Build history of the part. All positions in model axes, mm. Face numbers are marked on the shaded views. A direction names the side the tool comes from. Give positions to 0.01 mm unless a question says otherwise; leave off trailing zeros. Write each loop counter-clockwise with the first axis right and the second up, starting at its lowest first coordinate (ties: lowest second). Pieces come first, ordered by that corner, then holes. Notation, with made-up numbers: M 4.5,44 L 10.5,44 A19 cw 10.5,56 Z; hole C 77,66.5 d7. An arc over 180 degrees is marked long. One line per item, written item: value. Start each with the question number.
from build123d import *

# Parameters (mm, degrees)
SKETCH1_W           = 38
SKETCH1_H           = 30
SKETCH1_W_2         = 35
SKETCH1_H_2         = 27.631578948
BOSS_EXTRUDE1_DEPTH = 28.84
FILLET1_R           = 1
SKETCH2_W           = 35
SKETCH2_H           = 27.631578948
BOSS_EXTRUDE2_DEPTH = 3
SKETCH3_W           = 36.5
SKETCH3_H           = 28.815789474
CUT_EXTRUDE1_DEPTH  = 36.407705376
FILLET2_R           = 1


with BuildPart() as part:
    # Sketch1 → Boss-Extrude1 (new body)
    with BuildSketch(Plane.XY):
        Rectangle(SKETCH1_W, SKETCH1_H)
        Rectangle(SKETCH1_W_2, SKETCH1_H_2, mode=Mode.SUBTRACT)
    extrude(amount=BOSS_EXTRUDE1_DEPTH)

    # Fillet1
    fillet1_edges = [part.edges().sort_by_distance(p)[0] for p in [
        (19, 0, 28.84),
        (0, 15, 28.84),
        (-19, 0, 28.84),
        (0, -15, 28.84),
    ]]
    fillet(fillet1_edges, radius=FILLET1_R)

    # Sketch2 → Boss-Extrude2 (add)
    with BuildSketch(Plane(origin=(0, 0, 0), x_dir=(-1, 0, 0), z_dir=(0, 0, -1))):
        Rectangle(SKETCH2_W, SKETCH2_H)
    extrude(amount=-BOSS_EXTRUDE2_DEPTH)

    # Sketch3 → Cut-Extrude1 (cut, through all)
    with BuildSketch(Plane(origin=(0, 0, 3), x_dir=(-1, 0, 0), z_dir=(0, 0, -1))):
        with Locations((-0.75, -0.592105263)):
            Rectangle(SKETCH3_W, SKETCH3_H)
    extrude(amount=-CUT_EXTRUDE1_DEPTH, mode=Mode.SUBTRACT)

    # Fillet2
    # the kernel refuses this fillet: 1 mm, written as the material it takes off along each edge
    with BuildSketch(Plane(origin=(-18, -14, 27.84), x_dir=(-1, 0, 0), z_dir=(0, -1, 0))) as fillet2_piece_1_section:
        Polygon((0, 0), (FILLET2_R * 1.02, 0), (FILLET2_R * 1.02, -FILLET2_R * 1.02), (0, -FILLET2_R * 1.02), align=None)
    fillet2_piece_1 = extrude(amount=FILLET2_R * 1.02, mode=Mode.PRIVATE)
    fillet2_piece_1 = fillet2_piece_1 - Plane(origin=(-18, -14, 27.84), x_dir=(0.7071067811865475, 0, -0.7071067811865475), z_dir=(0, -1, 0)) * Sphere(FILLET2_R, mode=Mode.PRIVATE)
    add(fillet2_piece_1, mode=Mode.SUBTRACT)
    with BuildSketch(Plane(origin=(-18, 14, 27.84), x_dir=(-1, 0, 0), z_dir=(0, 1, 0))) as fillet2_piece_2_section:
        Polygon((0, 0), (FILLET2_R * 1.02, 0), (FILLET2_R * 1.02, FILLET2_R * 1.02), (0, FILLET2_R * 1.02), align=None)
    fillet2_piece_2 = extrude(amount=FILLET2_R * 1.02, mode=Mode.PRIVATE)
    fillet2_piece_2 = fillet2_piece_2 - Plane(origin=(-18, 14, 27.84), x_dir=(0.7071067811865475, 0, -0.7071067811865475), z_dir=(0, 1, 0)) * Sphere(FILLET2_R, mode=Mode.PRIVATE)
    add(fillet2_piece_2, mode=Mode.SUBTRACT)
    with BuildSketch(Plane(origin=(18, 14, 27.84), x_dir=(0, 1, 0), z_dir=(1, 0, 0))) as fillet2_piece_3_section:
        Polygon((0, 0), (FILLET2_R * 1.02, 0), (FILLET2_R * 1.02, FILLET2_R * 1.02), (0, FILLET2_R * 1.02), align=None)
    fillet2_piece_3 = extrude(amount=FILLET2_R * 1.02, mode=Mode.PRIVATE)
    fillet2_piece_3 = fillet2_piece_3 - Plane(origin=(18, 14, 27.84), x_dir=(0, -0.7071067811865475, -0.7071067811865475), z_dir=(1, 0, 0)) * Sphere(FILLET2_R, mode=Mode.PRIVATE)
    add(fillet2_piece_3, mode=Mode.SUBTRACT)
    with BuildSketch(Plane(origin=(18, -14, 1), x_dir=(1, 0, 0), z_dir=(0, -1, 0))) as fillet2_piece_4_section:
        Polygon((0, 0), (FILLET2_R * 1.02, 0), (FILLET2_R * 1.02, -FILLET2_R * 1.02), (0, -FILLET2_R * 1.02), align=None)
    fillet2_piece_4 = extrude(amount=FILLET2_R * 1.02, mode=Mode.PRIVATE)
    fillet2_piece_4 = fillet2_piece_4 - Plane(origin=(18, -14, 1), x_dir=(-0.7071067811865475, 0, 0.7071067811865475), z_dir=(0, -1, 0)) * Sphere(FILLET2_R, mode=Mode.PRIVATE)
    add(fillet2_piece_4, mode=Mode.SUBTRACT)
    with BuildSketch(Plane(origin=(18, -14, 2), x_dir=(1, 0, 0), z_dir=(0, -1, 0))) as fillet2_piece_5_section:
        Polygon((0, 0), (FILLET2_R * 1.02, 0), (FILLET2_R * 1.02, FILLET2_R * 1.02), (0, FILLET2_R * 1.02), align=None)
    fillet2_piece_5 = extrude(amount=FILLET2_R * 1.02, mode=Mode.PRIVATE)
    fillet2_piece_5 = fillet2_piece_5 - Plane(origin=(18, -14, 2), x_dir=(-0.7071067811865475, 0, -0.7071067811865475), z_dir=(0, -1, 0)) * Sphere(FILLET2_R, mode=Mode.PRIVATE)
    add(fillet2_piece_5, mode=Mode.SUBTRACT)
    with BuildSketch(Plane(origin=(19, 15, -2.5), x_dir=(0, -1, 0), z_dir=(0, 0, 1)), Plane(origin=(-19, 15, -2.5), x_dir=(1, 0, 0), z_dir=(0, 0, 1))) as fillet2_piece_6:
        with BuildLine():
            CenterArc((FILLET2_R, -FILLET2_R), FILLET2_R, 90, 90)
            Line((0, -FILLET2_R), (0, 0))
            Line((0, 0), (FILLET2_R, 0))
        make_face()
    extrude(amount=30.34, mode=Mode.SUBTRACT)
    with BuildSketch(Plane(origin=(-19, -15, -2.5), x_dir=(1, 0, 0), z_dir=(0, 0, 1))) as fillet2_piece_7:
        with BuildLine():
            CenterArc((FILLET2_R, FILLET2_R), FILLET2_R, 180, 90)
            Line((0, FILLET2_R), (0, 0))
            Line((0, 0), (FILLET2_R, 0))
        make_face()
    extrude(amount=30.34, mode=Mode.SUBTRACT)
    with BuildSketch(Plane(origin=(19, 17.5, 0), x_dir=(0, 0, 1), z_dir=(0, -1, 0))) as fillet2_piece_8:
        with BuildLine():
            CenterArc((FILLET2_R, FILLET2_R), FILLET2_R, 180, 90)
            Line((0, FILLET2_R), (0, 0))
            Line((0, 0), (FILLET2_R, 0))
        make_face()
    extrude(amount=31.5, mode=Mode.SUBTRACT)
    with BuildSketch(Plane(origin=(18, -15, 0), x_dir=(0, 0, 1), z_dir=(-1, 0, 0))) as fillet2_piece_9:
        with BuildLine():
            CenterArc((FILLET2_R, FILLET2_R), FILLET2_R, 180, 90)
            Line((0, FILLET2_R), (0, 0))
            Line((0, 0), (FILLET2_R, 0))
        make_face()
    extrude(amount=39.5, mode=Mode.SUBTRACT)
    with BuildSketch(Plane(origin=(19, -15, 1), x_dir=(-1, 0, 0), z_dir=(0, 0, 1))) as fillet2_piece_10:
        with BuildLine():
            CenterArc((FILLET2_R, -FILLET2_R), FILLET2_R, 90, 90)
            Line((0, -FILLET2_R), (0, 0))
            Line((0, 0), (FILLET2_R, 0))
        make_face()
    extrude(amount=1, mode=Mode.SUBTRACT)
    with BuildSketch(Plane(origin=(19, 13.815789474, 3), x_dir=(0, 0, -1), z_dir=(0, -1, 0))) as fillet2_piece_11:
        with BuildLine():
            CenterArc((FILLET2_R, -FILLET2_R), FILLET2_R, 90, 90)
            Line((0, -FILLET2_R), (0, 0))
            Line((0, 0), (FILLET2_R, 0))
        make_face()
    extrude(amount=27.815789474, mode=Mode.SUBTRACT)
    with BuildSketch(Plane(origin=(18, -15, 3), x_dir=(0, 0, -1), z_dir=(-1, 0, 0))) as fillet2_piece_12:
        with BuildLine():
            CenterArc((FILLET2_R, -FILLET2_R), FILLET2_R, 90, 90)
            Line((0, -FILLET2_R), (0, 0))
            Line((0, 0), (FILLET2_R, 0))
        make_face()
    extrude(amount=35.5, mode=Mode.SUBTRACT)


solid = part.part
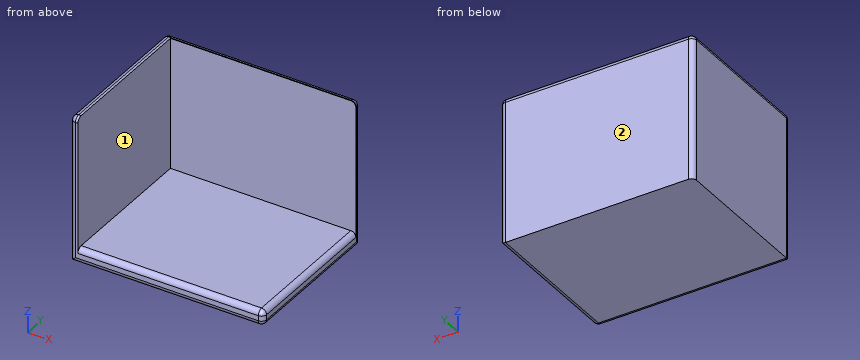
1) Band-saw the part on B-B (z = 15). List the corners of the cut face in (x, y).
2) Tool access for the marked faces 1 and 2: list every direction of +Z, -Z, +X, -X, +Y, -Y with a clear straight run to the whole face (end or side of a thin tool).
3) Probe line 1 along Y through (x, z) = (-8, 7.5); line 2 along Z through (x, y) = (15.5, -10.25); line 3 along X through (y, z) = (-4.25, 12). List the from-to ranges inside material, lowest first. Write a range as from..to.
4) Band-saw the part on A-A (y = -5.5). List the corners of the cut face in (x, z), then the cut area to 3 significant figures.
5) Drop flat-ended pins along their axis: P1, Ø3, axis at x = 14.5, z = 8, coming from the -Y side; P2, Ø10, axis at x = -4.5, y = 9, coming from the +Z side; P3, Ø3, axis at y = 0, z = 4, coming from the +X side; P4, Ø6, axis at y = -3, z = 25, coming from the +X side. Give the stop position or say it passes through.
Model answer:
1. outline: M -19,-14 A1 ccw -18,-15 L -17.5,-15 L -17.5,13.82 L 19,13.82 L 19,14 A1 ccw 18,15 L -18,15 A1 ccw -19,14 Z
2. face 1: +Z, +X, -Y
2. face 2: +Z, -Z, +X, -X, +Y
3. line 1: y = 13.82..15
3. line 2: z = 0..3
3. line 3: x = -19..-17.5
4. outline: M -19,0 L 18,0 A1 ccw 19,1 L 19,2 A1 ccw 18,3 L -17.5,3 L -17.5,28.84 L -18,28.84 A1 ccw -19,27.84 Z
4. area: 152 mm²
5. P1: stops at y = 13.82
5. P2: stops at z = 28.84
5. P3: stops at x = 18.87
5. P4: stops at x = -17.5
